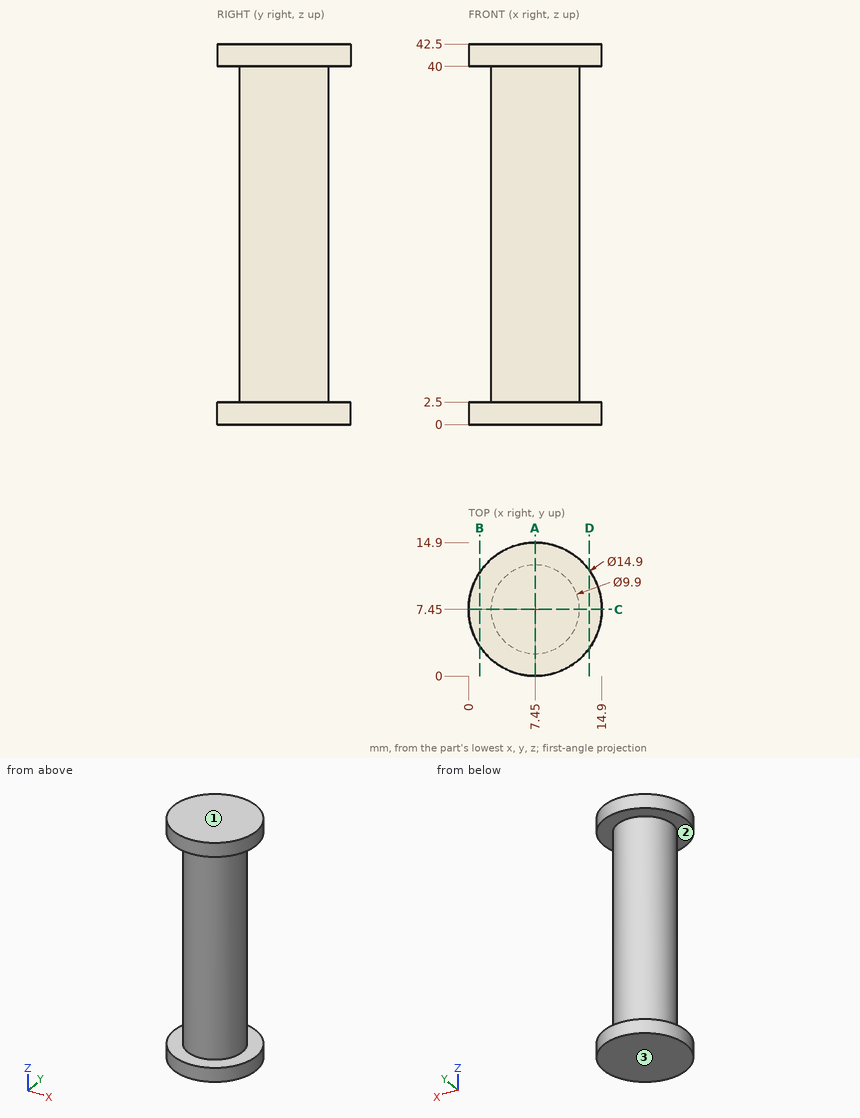
Check sheet for the drawn part. Datum: minimum x, y, z corner. Units: mm. Give positions to 0.01 mm unless a question says otherwise; leave off trailing zeros. Order: outer loops, then holes, each group sorted by start corner. A loop starts at its lowest first (then second) coordinate and runs counter-clockwise, first axis right, second up. Notation, with made-up numbers: (53.5, 30.5) - (63.5, 30.5) arc R36 cw to (63.5, 65.5) - close; hole circle Ø6 at (-20.75, 15). An arc over 180 degrees is marked (long way). Answer as a JSON object with one key per item and string values.
(1) Cross-section at D-D (x = 13.5). Record the cut outline in (y, z).
Report:
{"outline": "(3.1, 0) - (11.8, 0) - (11.8, 2.5) - (3.1, 2.5) - close; (3.1, 40) - (11.8, 40) - (11.8, 42.5) - (3.1, 42.5) - close"}
(2) Cross-section at A-A (x = 7.45). Record the cut outline in (y, z), then the cut area to 3 significant figures.
Report:
{"outline": "(0, 0) - (14.9, 0) - (14.9, 2.5) - (12.4, 2.5) - (12.4, 40) - (14.9, 40) - (14.9, 42.5) - (0, 42.5) - (0, 40) - (2.5, 40) - (2.5, 2.5) - (0, 2.5) - close", "area": "446 mm^2"}
(3) Draft check along Z on the marked faces 1, 2 and 3. Enter one of: released by +Z, released by -Z, zero draft, split by the parting line, or undercut.
Report:
{"face 1": "released by +Z", "face 2": "undercut", "face 3": "released by -Z"}
(4) Depth check by flat-ended pin: pin 1 Ø7.5 at (x, y) = (6, 9) entering from -Z; pin 2 Ø5 at (y, z) = (12, 22) entering from -X; pin 3 Ø6 at (x, z) = (9.5, 36.5) entering from -Y; pin 4 Ø3 at (y, z) = (10.5, 31.5) entering from +X. Enter the tip coordinate at first touch or a pass-through.
Report:
{"pin 1": "z = 0", "pin 2": "x = 2.94", "pin 3": "y = 2.5", "pin 4": "x = 12.15"}
(5) Material ranges on line 1 (Z direction, x = 3, y = 3.75); line 2 (X direction, y = 7.25, z = 15); line 3 (X direction, y = 8.75, z = 21), recorded low to high.
Report:
{"line 1": "0 to 2.5, 40 to 42.5", "line 2": "2.5 to 12.4", "line 3": "2.67 to 12.23"}
(6) Cross-section at B-B (x = 1.25). Record the cut outline in (y, z).
Report:
{"outline": "(3.32, 0) - (11.58, 0) - (11.58, 2.5) - (3.32, 2.5) - close; (3.32, 40) - (11.58, 40) - (11.58, 42.5) - (3.32, 42.5) - close"}
